CAD build for the part. Positions are in the model's coordinates, mm. Face numbers are marked on the shaded views. Coordinates: 2 decimals unless noted, no trailing zeros. Loops run counter-clockwise (first coordinate to the right, second up) from the corner with the lowest first, then second, coordinate; pieces in that order, holes last. Notation, with made-up numbers: (-11, -27) -> (43, -27) arc R13 ccw to (43, -14) -> close; hole circle Ø7 at (63.25, 68.25). An arc over 180 degrees is marked (long way). Write item = value, one per line. Start each with the question number.
(1) Drill centre lines: line 1 (Z direction, x = 27.5, y = 9.5); line 2 (Y direction, x = 25, z = -21.5); line 3 (Y direction, x = 20.5, z = 0.75). Where is each one in solid material? Low to high. Write a range as from..to.
(2) Band-saw the part on C-C (z = -20). Write the cut outline in (x, y).
(3) Band-saw the part on D-D (y = -140.5). Write the cut outline in (x, z).
(4) Band-saw the part on A-A (y = 39.5). Write the cut outline in (x, z).
(5) Band-saw the part on B-B (x = -39.5). Write the cut outline in (y, z), and give its area (4 significant figures).
(6) Pull direction X, two halves, no side cores. Call the marked faces 1 and 2: +X half, -X half, draft (parallel to the pull), parting line (faces both ways), or undercut.
(7) Flat gauge pins, fed straight in: P1, Ø2, axis at x = -22.5, y = 14.5, coming from the -Z side; P2, Ø4, axis at x = 21, z = -13.5, coming from the -Y side; P3, Ø15, axis at x = 6, z = -3.5, coming from the +Y side. Where does each tip first touch, or does it go through?
Autodesk Inventor part; units mm, degrees
ref_plane "YZ Plane" through (0, 0, 0) normal (1, 0, 0) x (0, 1, 0)
ref_plane "XZ Plane" through (0, 0, 0) normal (0, 1, 0) x (-1, 0, 0)
ref_plane "XY Plane" through (0, 0, 0) normal (0, 0, 1) x (1, 0, 0)
sketch "Sketch1" plane through (0, 0, 0) normal (0, 0, 1) x (1, 0, 0)
  line L0 (-50, -100) -> (50, -100)
  line L1 (50, -100) -> (50, 100)
  line L2 (50, 100) -> (-50, 100)
  line L3 (-50, 100) -> (-50, -100)
  line L4 (-50, -100) -> (50, 100) construction
  line L5 (50, -100) -> (-50, 100) construction
  point P0 (0, 0)
  dimension "d0" = 100
  dimension "d1" = 200
extrude "Extrusion1" add sketch "Sketch1" along normal blind 5
sketch "Sketch6" plane through (0, 0, 5) normal (0, 0, 1) x (1, 0, 0)
  line L0 (4.9986, 75) -> (-5.0014, 75)
  line L1 (-25.0014, 55) -> (-25.0014, 45)
  line L2 (-5.0014, 25) -> (4.9986, 25)
  line L3 (24.9986, 45) -> (24.9986, 55)
  line L4 (24.9986, 75) -> (-25.0014, 25) construction
  line L5 (-25.0014, 75) -> (24.9986, 25) construction
  arc A0 (4.9986, 25) -> (24.9986, 45) centre (4.9986, 45) ccw
  arc A1 (24.9986, 55) -> (4.9986, 75) centre (4.9986, 55) ccw
  arc A2 (-5.0014, 75) -> (-25.0014, 55) centre (-5.0014, 55) ccw
  arc A3 (-25.0014, 45) -> (-5.0014, 25) centre (-5.0014, 45) ccw
  point P0 (0, 0)
  point P1 (-0.0014, 50)
  dimension "d21" = 50
  dimension "d22" = 50
  dimension "d23" = 20
extrude "Extrusion6" cut sketch "Sketch6" against normal blind 5
sketch "Sketch15" plane through (-50, 100, 5) normal (0, 1, 0) x (1, 0, 0)
  line L0 (100, 0) -> (0, 0)
  line L1 (0, 0) -> (100, 0)
  line L2 (100, 0) -> (100, 30)
  line L3 (100, 30) -> (0, 30)
  line L4 (0, 30) -> (0, 0)
  point P0 (50, 5)
  dimension "d46" = 100
  dimension "d47" = 30
sketch "Sketch16" plane through (-50, 100, 5) normal (0, 1, 0) x (1, 0, 0)
  circle A0 centre (10.5, 5) radius 4.5
  circle A1 centre (89.5, 5) radius 4.5
  circle A2 centre (10.5, 25) radius 4.5
  circle A3 centre (89.5, 25) radius 4.5
  point P0 (50, 5)
  dimension "d48" = 9
  dimension "d49" = 9
  dimension "d50" = 9
  dimension "d51" = 9
extrude "Extrusion11" add sketch "Sketch15" against normal blind 5
extrude "Extrusion12" add sketch "Sketch16" along normal blind 15
sketch "Sketch21" plane through (0, 0, 5) normal (0, 0, 1) x (1, 0, 0)
  line L0 (50, -100) -> (50, 100)
  line L1 (50, -100) -> (-50, -100)
  line L2 (-50, -100) -> (-50, -180)
  line L3 (-50, -180) -> (50, -180)
  line L4 (50, -180) -> (50, -100)
  point P0 (0, 0)
  dimension "d66" = 100
  dimension "d67" = 80
extrude "Extrusion17" add sketch "Sketch21" against normal blind 5
properties part number "fixation_v04"
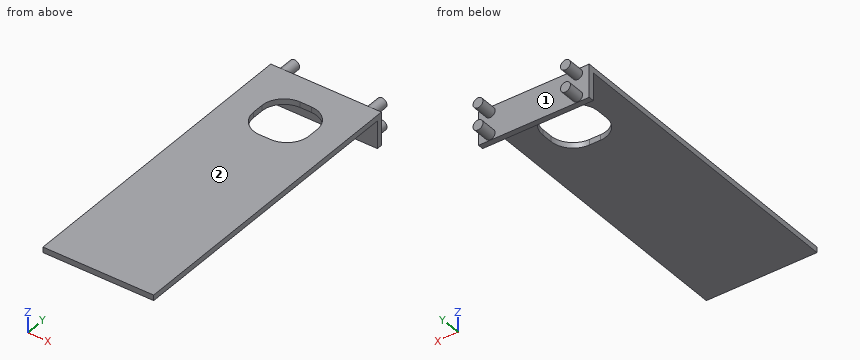
Findings below:
q1.line_1 = 0..5
q1.line_2 = 95..100
q1.line_3 = -180..32.36, 67.64..100
q2.outline = (-50, 95) -> (50, 95) -> (50, 100) -> (44, 100) -> (44, 115) -> (35, 115) -> (35, 100) -> (-35, 100) -> (-35, 115) -> (-44, 115) -> (-44, 100) -> (-50, 100) -> close
q3.outline = (-50, 0) -> (50, 0) -> (50, 5) -> (-50, 5) -> close
q4.outline = (-50, 0) -> (-24.23, 0) -> (-24.23, 5) -> (-50, 5) -> close; (24.23, 0) -> (50, 0) -> (50, 5) -> (24.23, 5) -> close
q5.outline = (-180, 0) -> (95, 0) -> (95, -25) -> (100, -25) -> (100, -24.5) -> (115, -24.5) -> (115, -15.5) -> (100, -15.5) -> (100, -4.5) -> (115, -4.5) -> (115, 4.5) -> (100, 4.5) -> (100, 5) -> (-180, 5) -> close
q5.area = 1,795 mm²
q6.face_1 = undercut
q6.face_2 = draft
q7.P1 = 0
q7.P2 = 95
q7.P3 = 100
